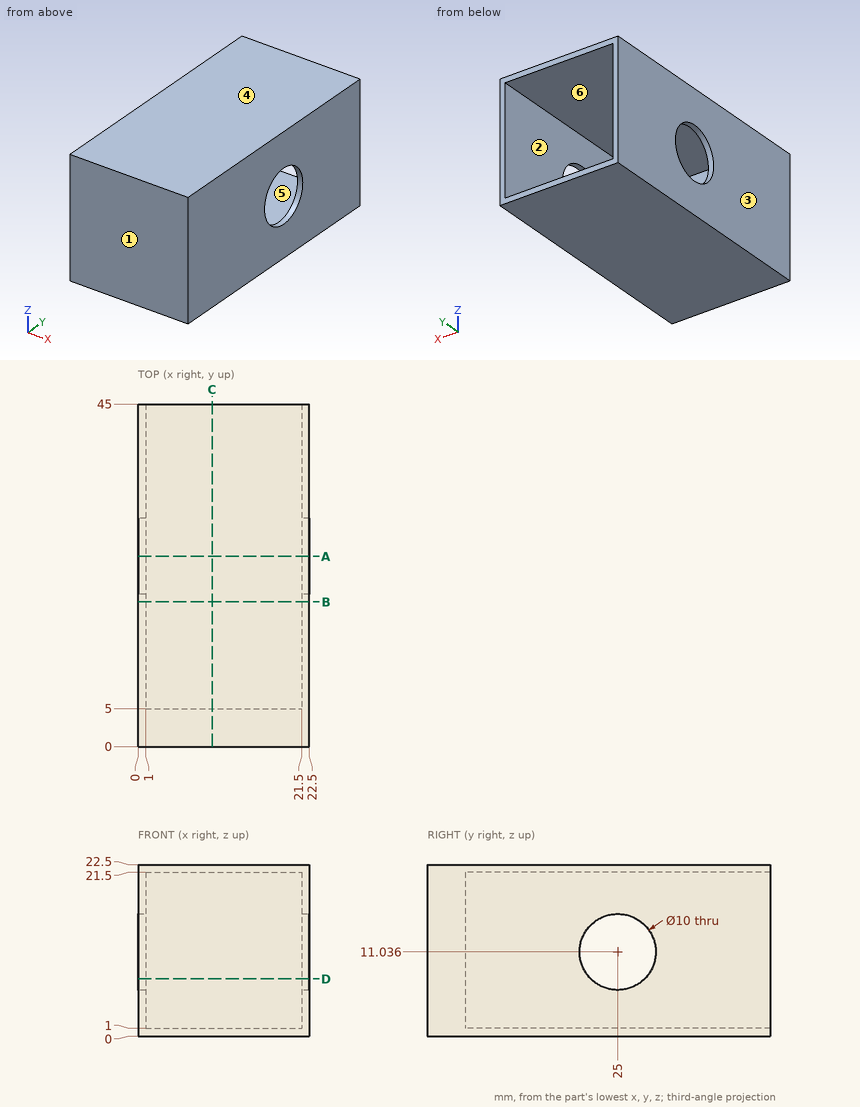
Can you work these out from the drawing? Everything is in mm from the part's minimum corner. A direction names the side the tool comes from. Give positions to 0.01 mm unless a question says otherwise; leave off trailing zeros. Loops run counter-clockwise (first coordinate to the right, second up) from the corner with the lowest first, then second, coordinate; pieces in that order, holes last. Notation, with made-up numbers: (32, -16) - (76, -16) arc R28 cw to (76, 5) - close; hole circle Ø9 at (52.25, -12). An arc over 180 degrees is marked (long way). Answer as a JSON object with one key per item and string values.
Q1. Which directions (+Z, -Z, +X, -X, +Y, -Y) give clear straight access to the entire face, cutting with the end or side of a thin tool? Please do the marked faces 1 and 2.
Geometry says:
{"face 1": "+Z, -Z, +X, -X, -Y", "face 2": "+Y"}
Q2. Imagine slicing it at C-C on x = 9.75. Write out the boundary of the cut face in (y, z), plus the area to 4 significant figures.
Geometry says:
{"outline": "(0, 0) - (45, 0) - (45, 1) - (5, 1) - (5, 21.5) - (45, 21.5) - (45, 22.5) - (0, 22.5) - close", "area": "192.5 mm²"}
Q3. Imagine slicing it at A-A on y = 25. Write out the boundary of the cut face in (x, z), plus the area to 3 significant figures.
Geometry says:
{"outline": "(0, 0) - (22.5, 0) - (22.5, 6.04) - (21.5, 6.04) - (21.5, 1) - (1, 1) - (1, 6.04) - (0, 6.04) - close; (0, 16.04) - (1, 16.04) - (1, 21.5) - (21.5, 21.5) - (21.5, 16.04) - (22.5, 16.04) - (22.5, 22.5) - (0, 22.5) - close", "area": "66.0 mm²"}
Q4. Will these pins go through, and if not, where does the flat tip stop? P1, Ø6, axis at y = 25, z = 11.04, coming from the -X side; P2, Ø10, axis at x = 6.5, z = 11.5, coming from the +Y side.
Geometry says:
{"P1": "through", "P2": "y = 5"}
Q5. Imagine slicing it at D-D on z = 7.5. Write out the boundary of the cut face in (x, y) (3 decimals).
Geometry says:
{"outline": "(0, 0) - (22.5, 0) - (22.5, 21.465) - (21.5, 21.465) - (21.5, 5) - (1, 5) - (1, 21.465) - (0, 21.465) - close; (0, 28.535) - (1, 28.535) - (1, 45) - (0, 45) - close; (21.5, 28.535) - (22.5, 28.535) - (22.5, 45) - (21.5, 45) - close"}
Q6. If I drill on L1, parallel to X at y = 31, z = 7.25; L2, parallel to Y at x = 1.5, z = 13.5, over which ranges is the centre line in solid material (lowest first)?
Geometry says:
{"L1": "0 to 1, 21.5 to 22.5", "L2": "0 to 5"}
Q7. If we mould it in two halves opening along X, with no side actions, what happens to the marked faces 3, 4, 5 and 6? For each: pulls with the +X half, pulls with the -X half, needs draft (parallel to the pull), parting line crosses it, or undercut.
Geometry says:
{"face 3": "pulls with the -X half", "face 4": "needs draft", "face 5": "undercut", "face 6": "undercut"}
Q8. Imagine slicing it at B-B on y = 19. Write out the boundary of the cut face in (x, z), plus the area to 3 significant figures.
Geometry says:
{"outline": "(0, 0) - (22.5, 0) - (22.5, 22.5) - (0, 22.5) - close; hole (1, 1) - (21.5, 1) - (21.5, 21.5) - (1, 21.5) - close", "area": "86.0 mm²"}
